from build123d import *

# Parameters (mm, degrees)
SKETCH1_W           = 50.8
SKETCH1_H           = 50.8
BOSS_EXTRUDE1_DEPTH = 3
BOSS_EXTRUDE2_DEPTH = 5
FILLET1_R           = 2
SKETCH3_R           = 3.302
CUT_EXTRUDE3_DEPTH  = 75.162524229
FILLET2_R           = 2.54


with BuildPart() as part:
    # Sketch1 → Boss-Extrude1 (new body)
    with BuildSketch(Plane.XY):
        with Locations((25.4, 25.4)):
            Rectangle(SKETCH1_W, SKETCH1_H)
    extrude(amount=BOSS_EXTRUDE1_DEPTH)

    # Sketch8 → Boss-Extrude2 (add)
    with BuildSketch(Plane(origin=(3, 0, 3), x_dir=(1, 0, 0), z_dir=(0, 0, 1))):
        with BuildLine():
            Line((14.4, 9.95), (14.4, 16.117488447))
            ThreePointArc((14.4, 16.117488447), (14.028025612, 17.015514059), (13.13, 17.387488447))
            Line((13.13, 17.387488447), (6.962511553, 17.387488447))
            Line((6.962511553, 17.387488447), (0.2, 24.15))
            Line((0.2, 24.15), (0.2, 26.65))
            Line((0.2, 26.65), (7.217411382, 33.667411382))
            Line((7.217411382, 33.667411382), (13.384899829, 33.667411382))
            ThreePointArc((13.384899829, 33.667411382), (14.282925441, 34.03938577), (14.654899829, 34.937411382))
            Line((14.654899829, 34.937411382), (14.654899829, 41.104899829))
            Line((14.654899829, 41.104899829), (21.15, 47.6))
            Line((21.15, 47.6), (23.65, 47.6))
            Line((23.65, 47.6), (30.667411382, 40.582588618))
            Line((30.667411382, 40.582588618), (30.667411382, 34.415100171))
            ThreePointArc((30.667411382, 34.415100171), (31.03938577, 33.517074559), (31.937411382, 33.145100171))
            Line((31.937411382, 33.145100171), (38.104899829, 33.145100171))
            Line((38.104899829, 33.145100171), (44.6, 26.65))
            Line((44.6, 26.65), (44.6, 24.15))
            Line((44.6, 24.15), (37.824884254, 17.374884254))
            Line((37.824884254, 17.374884254), (31.657395807, 17.374884254))
            ThreePointArc((31.657395807, 17.374884254), (30.759370195, 17.002909866), (30.387395807, 16.104884254))
            Line((30.387395807, 16.104884254), (30.387395807, 9.937395807))
            Line((30.387395807, 9.937395807), (23.65, 3.2))
            Line((23.65, 3.2), (21.15, 3.2))
            Line((21.15, 3.2), (14.4, 9.95))
        make_face()
    extrude(amount=BOSS_EXTRUDE2_DEPTH)

    # Fillet1
    fillet1_edges = [part.edges().sort_by_distance(p)[0] for p in [
        (17.4, 9.95, 5.5),
        (24.15, 3.2, 5.5),
        (26.65, 3.2, 5.5),
        (33.387395807, 9.937395807, 5.5),
        (40.824884254, 17.374884254, 5.5),
        (47.6, 24.15, 5.5),
        (47.6, 26.65, 5.5),
        (41.104899829, 33.145100171, 5.5),
        (33.667411382, 40.582588618, 5.5),
        (26.65, 47.6, 5.5),
        (24.15, 47.6, 5.5),
        (17.654899829, 41.104899829, 5.5),
        (10.217411382, 33.667411382, 5.5),
        (3.2, 26.65, 5.5),
        (3.2, 24.15, 5.5),
        (9.962511553, 17.387488447, 5.5),
    ]]
    fillet(fillet1_edges, radius=FILLET1_R)

    # Sketch3 → Cut-Extrude3 (cut, through all)
    with BuildSketch(Plane(origin=(-3, 0, 3), x_dir=(-1, 0, 0), z_dir=(0, 0, -1))):
        with Locations((-15.7, 12.7)):
            Circle(SKETCH3_R)
        with Locations((-41.1, 38.1)):
            Circle(SKETCH3_R)
        with Locations((-15.7, 38.1)):
            Circle(SKETCH3_R)
        with Locations((-41.1, 12.7)):
            Circle(SKETCH3_R)
    extrude(amount=CUT_EXTRUDE3_DEPTH, mode=Mode.SUBTRACT)

    # Fillet2
    fillet2_edges = [part.edges().sort_by_distance(p)[0] for p in [
        (0, 50.8, 1.5),
        (50.8, 50.8, 1.5),
        (50.8, 0, 1.5),
        (0, 0, 1.5),
    ]]
    fillet(fillet2_edges, radius=FILLET2_R)


solid = part.part
Build history of the part. All positions in model axes, mm. A direction names the side the tool comes from. Give positions to 0.01 mm unless a question says otherwise; leave off trailing zeros. Order: outer loops, then holes, each group sorted by start corner. A loop starts at its lowest first (then second) coordinate and runs counter-clockwise, first axis right, second up. Notation, with made-up numbers: M 87,22 L 103,22 A27 cw 103,48 Z; hole C 11.5,50 d11. An arc over 180 degrees is marked long. Use one line per item in the form item = value.
1) Drop flat-ended pins along their axis: pin 1 (1.5 mm diameter, centred on x = 10.5, y = 15.5, fed in from -Z); pin 2 (1 mm diameter, centred on x = 21, z = 5.5, fed in from -Y); pin 3 (7.5 mm diameter, centred on x = 12.7, y = 12.7, fed in from +Z); pin 4 (2.5 mm diameter, centred on y = 13.5, z = 5, fed in from +X). Give the stop position or say it passes through.
Calculated:
pin_1 = 0
pin_2 = 5.85
pin_3 = 3
pin_4 = 33.39
2) Saw through at B-B (x = 12.7). Give the cut face in (y, z), plus the area to 3 significant figures.
Calculated:
outline = M 0,0 L 9.4,0 L 9.4,3 L 0,3 Z; M 16,0 L 34.8,0 L 34.8,3 L 33.67,3 L 33.67,8 L 17.39,8 L 17.39,3 L 16,3 Z; M 41.4,0 L 50.8,0 L 50.8,3 L 41.4,3 Z
area = 194 mm2
3) Two-plate mould, pull along Y, no slides. Class faces 5 (the face through (41.4, 38.2, 1.5)), 6 (the face through (17.4, 13, 5)), 7 (the face through (3.35, 24.22, 5.54)): released by +Y, released by -Y, zero draft, split by the parting line, or undercut.
Calculated:
face_5 = undercut
face_6 = zero draft
face_7 = released by -Y
4) Saw through at D-D (y = 31.5). Give the cut face in (x, z), plus the area to 3 significant figures.
Calculated:
outline = M 0,0 L 50.8,0 L 50.8,3 L 42.75,3 L 42.75,8 L 8.05,8 L 8.05,3 L 0,3 Z
area = 326 mm2
5) Probe probe 1 along Y at (x, z) = (38.1, 0.9); probe 2 along Z at (x, y) = (16, 10). List the from-to ranges inside material, lowest first.
Calculated:
probe_1 = 0 to 9.4, 16 to 34.8, 41.4 to 50.8
probe_2 = 0 to 3
6) Saw through at A-A (y = 12.7). Give the cut face in (x, z), plus the area to 3 significant figures.
Calculated:
outline = M 0,0 L 9.4,0 L 9.4,3 L 0,3 Z; M 16,0 L 34.8,0 L 34.8,3 L 33.39,3 L 33.39,8 L 17.4,8 L 17.4,3 L 16,3 Z; M 41.4,0 L 50.8,0 L 50.8,3 L 41.4,3 Z
area = 193 mm2
7) Tool access for faces 1 (the face through (34.03, 33.527, 5.465)), 2 (the face through (17.556, 10.003, 5.535)), 3 (the face through (36, 9, 3)), 4 (the face through (26.58, 3.35, 5.54)): list every direction of +Z, -Z, +X, -X, +Y, -Y with a clear straight run to the whole face (end or side of a thin tool).
Calculated:
face_1 = +Z, +X, +Y
face_2 = +Z, -X, -Y
face_3 = +Z
face_4 = +Z, +X, -Y
8) Saw through at C-C (x = 6.5). Give the cut face in (y, z), plus the area to 3 significant figures.
Calculated:
outline = M 0,0 L 50.8,0 L 50.8,3 L 29.95,3 L 29.95,8 L 20.85,8 L 20.85,3 L 0,3 Z
area = 198 mm2
